CAD build for the part. Positions are in the model's coordinates, mm. A direction names the side the tool comes from. Coordinates: 2 decimals unless noted, no trailing zeros. Order: outer loops, then holes, each group sorted by start corner. A loop starts at its lowest first (then second) coordinate and runs counter-clockwise, first axis right, second up. Notation, with made-up numbers: (34.5, 51.25) - (76.5, 51.25) arc R27 cw to (76.5, 82.25) - close; hole circle Ø7 at (61.25, 6). An arc over 180 degrees is marked (long way). Write each question's results on one line, items separated by ' | '. Start each with the question number.
Q1. Which spindle directions (+Z, -Z, +X, -X, +Y, -Y) get a long thin tool onto all of the face, cutting with end or side? Do faces 1 (the flat face through (625, 18, 2)), 2 (the flat face through (313, 11, 3)). Say none if no direction does.
Q2. Band-saw the part on B-B, the plane x = 531.5. Write the cut outline in (y, z), then the cut area to 3 significant figures.
Q3. Band-saw the part on C-C, the plane z = 11. Write the cut outline in (x, y).
Q4. Pin check, flat tips, straight feed: P1, Ø3, axis at y = 18.5, z = 3.5, coming from the -X side; P2, Ø6.5, axis at x = 369, z = 16, coming from the -Y side; P3, Ø4, axis at y = 21, z = 22, coming from the -X side. Stop position of each tip, or through.
Q5. Wall check: probe 1 along Y at (x, z) = (591.5, 4.5); probe 2 along Z at (x, y) = (560, 1.75); probe 3 along X at (y, z) = (23.25, 12.75). Give the ranges that are in metal, low to high.
Q6. Band-saw the part on A-A, the plane y = 8.75. Write the cut outline in (x, z), then the cut area to 3 significant figures.
```python
from build123d import *

# Parameters (mm, degrees)
F1_DEPTH    = 634
F2_T1_DEPTH = 47.7168298797
F4_DEPTH    = 25


# Not quite as in the source:
# - a fillet or chamfer that OpenCascade refuses, or shapes differently, is made with other operations: its cross-section is extruded or revolved along the edge and cut away or added


with BuildPart() as f1:
    # F0 (on Right) → F1 (new body)
    with BuildSketch(Plane.YZ):
        Polygon((0, 3), (0, 0), (25, 0), (25, 25), (22, 25), (22, 3), align=None)
    extrude(amount=F1_DEPTH)

    # F2: chamfer of 5 on 2 edges, made by hand

    # F2_s2 → F2_t1 (cut)
    with BuildSketch(Plane.XY.offset(-9.8584149398)):
        Polygon((629, 22), (634, 27), (634, 22), align=None)
        Polygon((5, 22), (0, 27), (0, 22), align=None)
    extrude(amount=F2_T1_DEPTH, mode=Mode.SUBTRACT)

    # F3 (on face) → F4 (cut)
    with BuildSketch(Plane.XY.offset(3)):
        Polygon((634, 22), (629, 22), (607, 0), (634, 0), align=None)
        Polygon((27, 0), (5, 22), (0, 22), (0, 0), align=None)
    extrude(amount=-F4_DEPTH, mode=Mode.SUBTRACT)


solid = f1.part
```
Results below:
1) face 1: +Z, -Z, +X, -Y | face 2: +Z, +X, -X, -Y
2) outline: (0, 0) - (25, 0) - (25, 25) - (22, 25) - (22, 3) - (0, 3) - close | area: 141 mm²
3) outline: (2, 25) - (5, 22) - (629, 22) - (632, 25) - close
4) P1: stops at x = 7.09 | P2: stops at y = 22 | P3: stops at x = 4
5) probe 1: y = 22 to 25 | probe 2: z = 0 to 3 | probe 3: x = 3.75 to 630.25
6) outline: (18.25, 0) - (615.75, 0) - (615.75, 3) - (18.25, 3) - close | area: 1,790 mm²
